The model under review builds one solid part; all positions refer to its coordinate system, in mm. Face numbers are marked on the shaded views. A direction names the side the tool comes from. Coordinates: 2 decimals unless noted, no trailing zeros. Loops run counter-clockwise (first coordinate to the right, second up) from the corner with the lowest first, then second, coordinate; pieces in that order, holes last. Notation, with made-up numbers: M 37,85.25 L 66,85.25 A35 ccw 66,119.25 Z; hole C 57,78.5 d5. An arc over 180 degrees is marked long. Return JSON: item names as keys, results as strings.
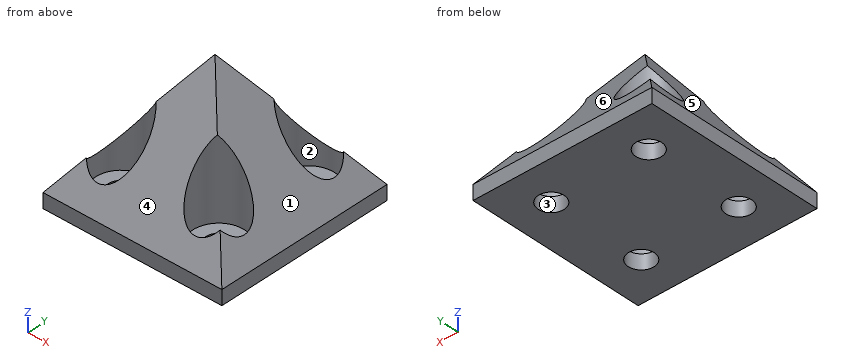
```python
from build123d import *

# Parameters (mm, degrees)
F0_W           = 36.7
F0_H           = 36.7
F0_R           = 5.25
F0_R_2         = 2.65
F1_DEPTH       = 25
F3_DEPTH       = 36.701
F5_DEPTH       = 43.2
F6_DEPTH       = 3
F9_D           = 5.3
F9_DEPTH       = 55
F9_CBORE_D     = 10.5
F9_CBORE_DEPTH = 50
F9_TIP         = 1.5922806404


with BuildPart() as f1:
    # F0 (on Top) → F1 (new body)
    with BuildSketch(Plane.XY):
        with Locations((-2.6058288604, -28.3063627124)):
            Rectangle(F0_W, F0_H)
        with Locations((-12.6058288604, -38.3063627124)):
            Circle(F0_R, mode=Mode.SUBTRACT)
        with Locations((7.3941711396, -38.3063627124)):
            Circle(F0_R, mode=Mode.SUBTRACT)
        with Locations((-12.6058288604, -18.3063627124)):
            Circle(F0_R, mode=Mode.SUBTRACT)
        with Locations((7.3941711396, -18.3063627124)):
            Circle(F0_R, mode=Mode.SUBTRACT)
        with Locations((-12.6058288604, -38.3063627124)):
            Circle(F0_R)
        with Locations((-12.6058288604, -38.3063627124)):
            Circle(F0_R_2, mode=Mode.SUBTRACT)
        with Locations((-12.6058288604, -38.3063627124)):
            Circle(F0_R_2)
        with Locations((7.3941711396, -38.3063627124)):
            Circle(F0_R)
        with Locations((7.3941711396, -38.3063627124)):
            Circle(F0_R_2, mode=Mode.SUBTRACT)
        with Locations((7.3941711396, -38.3063627124)):
            Circle(F0_R_2)
        with Locations((7.3941711396, -18.3063627124)):
            Circle(F0_R)
        with Locations((7.3941711396, -18.3063627124)):
            Circle(F0_R_2, mode=Mode.SUBTRACT)
        with Locations((7.3941711396, -18.3063627124)):
            Circle(F0_R_2)
        with Locations((-12.6058288604, -18.3063627124)):
            Circle(F0_R)
        with Locations((-12.6058288604, -18.3063627124)):
            Circle(F0_R_2, mode=Mode.SUBTRACT)
        with Locations((-12.6058288604, -18.3063627124)):
            Circle(F0_R_2)
    extrude(amount=F1_DEPTH)

    # F2 (on face) → F3 (cut, through all)
    with BuildSketch(Plane.XZ.offset(46.6563627124)):
        Polygon((-20.9558288604, 0), (-2.6058288604, 25), (-20.9558288604, 25), align=None)
        Polygon((15.7441711396, 25), (-2.6058288604, 25), (15.7441711396, 0), align=None)
    extrude(amount=-F3_DEPTH, mode=Mode.SUBTRACT)

    # F4 (on Right) → F5 (cut, symmetric)
    with BuildSketch(Plane.YZ):
        Polygon((-46.6563627124, 0), (-28.3063627124, 25), (-46.6563627124, 25), align=None)
        Polygon((-9.9563627124, 25), (-28.3063627124, 25), (-9.9563627124, 0), align=None)
    extrude(amount=F5_DEPTH, both=True, mode=Mode.SUBTRACT)

    # F6 (add): a face of the model
    f6_faces = [f1.faces().sort_by_distance(p)[0] for p in [
        (-2.6058288604, -28.3063627124, 0),
    ]]
    extrude(f6_faces, amount=F6_DEPTH)

    # F9
    with Locations(Plane.XY.offset(50)):
        with Locations((-12.6058288604, -38.3063627124), (-12.6058288604, -18.3063627124), (7.3941711396, -18.3063627124), (7.3941711396, -38.3063627124)):
            CounterBoreHole(F9_D / 2, F9_CBORE_D / 2, F9_CBORE_DEPTH, depth=F9_DEPTH)
            with Locations((0, 0, -(F9_DEPTH + F9_TIP / 2))):  # 118° drill point
                Cone(0, F9_D / 2, F9_TIP, mode=Mode.SUBTRACT)


solid = f1.part
```
1. To check wall thickness, follow line 1 (X direction, y = -40, z = -0.5); line 2 (Z direction, x = -8, y = -17.5); line 3 (Y direction, x = -0.5, z = 11.5). State the ranges of each line that lie inside material, in increasing order.
Check values:
{"line 1": "-20.96 to -14.64, -10.57 to 5.36, 9.43 to 15.74", "line 2": "-3 to 0", "line 3": "-38.22 to -18.4"}
2. Add section A-A on x = -13. Give the boundary of the cut face in (y, z), plus the area to 3 significant figures.
Check values:
{"outline": "M -46.66,-3 L -40.93,-3 L -40.93,0 L -43.54,0 L -43.54,4.24 L -46.66,0 Z; M -35.69,-3 L -20.93,-3 L -20.93,0 L -23.54,0 L -23.54,10.84 L -33.07,10.84 L -33.07,0 L -35.69,0 Z; M -15.69,-3 L -9.96,-3 L -9.96,0 L -13.07,4.24 L -13.07,0 L -15.69,0 Z", "area": "195 mm²"}
3. Add section C-C on x = -6.5. Give the boundary of the cut face in (y, z).
Check values:
{"outline": "M -46.66,-3 L -9.96,-3 L -9.96,0 L -24.41,19.69 L -32.2,19.69 L -46.66,0 Z"}
4. The part is to be moulded in two halves that separate along Y. For the marked faces 3, 4, 5 and 6, say which applies: released by +Y, released by -Y, zero draft, split by the parting line, or undercut.
Check values:
{"face 3": "undercut", "face 4": "released by -Y", "face 5": "zero draft", "face 6": "released by +Y"}
5. Add section D-D on z = 15.75. Give the boundary of the cut face in (x, y).
Check values:
{"outline": "M -9.4,-34.15 A5.25 cw -8.45,-35.1 L 3.24,-35.1 A5.25 cw 4.18,-34.15 L 4.18,-22.46 A5.25 cw 3.24,-21.52 L -8.45,-21.52 A5.25 cw -9.4,-22.46 Z"}
6. Machinability: for the marked faces 1 and 2, which of the approach directions +Z, -Z, +X, -X, +Y, -Y give a long, thin tool a straight path to every point of the face, cutting with its end or side? Answer none if there is none.
Check values:
{"face 1": "+Z, +X, +Y, -Y", "face 2": "+Z"}
7. Insertion check: pin 1 Ø17 at (x, y) = (7.39, -38.31) entering from -Z; pin 2 Ø6 at (y, z) = (-31, 15.5) entering from +X; pin 3 Ø5 at (y, z) = (-20.5, 8) entering from +X; pin 4 Ø8 at (y, z) = (-21.5, 13.5) entering from +X. Each pin has a flat end and moves straight along its axis. Give the tip position at first contact, or say it passes through.
Check values:
{"pin 1": "z = -3", "pin 2": "x = 6.57", "pin 3": "x = 11.55", "pin 4": "x = 8.39"}
8. Add section B-B on y = -31. Give the boundary of the cut face in (x, z).
Check values:
{"outline": "M -20.96,-3 L 15.74,-3 L 15.74,0 L 0.09,21.33 L -5.3,21.33 L -20.96,0 Z"}
